from build123d import *

# Parameters (mm, degrees)
F0_W      = 100
F0_H      = 100
F1_DEPTH  = 20
F2_W      = 100
F2_H      = 80
F3_DEPTH  = 20
F4_W      = 30
F4_H      = 80
F5_DEPTH  = 80
F6_R      = 20
F7_R      = 15
F8_DEPTH  = 20
F9_W      = 40
F9_H      = 40
F10_DEPTH = 20
F11_SIZE  = 79.99999


# Not quite as in the source:
# - a fillet or chamfer is up to 0.001 mm smaller than in the source, because OpenCascade refuses the exact size


with BuildPart() as f1:
    # F0 (on Top) → F1 (new body)
    with BuildSketch(Plane.XY):
        with Locations((0.1719114778, -50)):
            Rectangle(F0_W, F0_H)
    extrude(amount=F1_DEPTH)

    # F2 (on Front) → F3 (join)
    with BuildSketch(Plane.XZ):
        with Locations((0.1466497779, 59.8839402659)):
            Rectangle(F2_W, F2_H)
    extrude(amount=F3_DEPTH)

    # F4 (on face) → F5 (join)
    with BuildSketch(Plane.XY.offset(20)):
        with Locations((35.1466497779, -60)):
            Rectangle(F4_W, F4_H)
    extrude(amount=F5_DEPTH)

    # F6
    f6_edges = [f1.edges().sort_by_distance(p)[0] for p in [
        (-49.828089, -100, 10),
    ]]
    fillet(f6_edges, radius=F6_R)

    # F7 (on face) → F8 (cut)
    with BuildSketch(Plane.XY.offset(20)):
        with Locations((-25.480100885, -75)):
            Circle(F7_R)
    extrude(amount=-F8_DEPTH, mode=Mode.SUBTRACT)

    # F9 (on face) → F10 (cut)
    with BuildSketch(Plane.XZ.offset(20)):
        with Locations((-13.2386269793, 61.6098302603)):
            Rectangle(F9_W, F9_H)
    extrude(amount=-F10_DEPTH, mode=Mode.SUBTRACT)

    # F11 (size 80 in the source; OpenCascade refuses exactly that, so slightly less here)
    f11_edges = [f1.edges().sort_by_distance(p)[0] for p in [
        (35.14665, -100, 100),
    ]]
    chamfer(f11_edges, length=F11_SIZE)


solid = f1.part
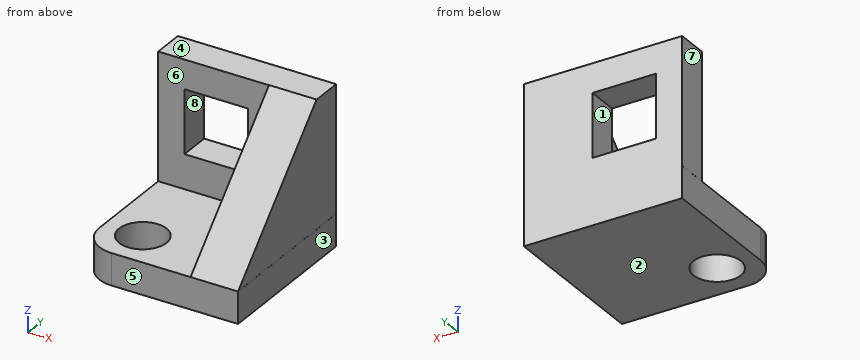
Part model, mm, in its own coordinate system. Face numbers are marked on the shaded views. A direction names the side the tool comes from. Coordinates: 2 decimals unless noted, no trailing zeros. Order: outer loops, then holes, each group sorted by start corner. A loop starts at its lowest first (then second) coordinate and runs counter-clockwise, first axis right, second up.
(1) Pin check, flat tips, straight feed: pin 1 Ø8 at (y, z) = (-87, 19) entering from -X; pin 2 Ø10 at (x, z) = (-36.5, 47) entering from -Y; pin 3 Ø1 at (x, y) = (37, -77) entering from +Z. Stop position of each tip, or through.
Check sheet entries:
pin 1: stops at x = -49.6
pin 2: stops at y = -20
pin 3: stops at z = 43.5
(2) Tool access for the marked faces 4, 5, 6, 7 and 8: list every direction of +Z, -Z, +X, -X, +Y, -Y with a clear straight run to the whole face (end or side of a thin tool).
Check sheet entries:
face 4: +Z, +X, -X, +Y
face 5: +Z, -Z, +X, -X, -Y
face 6: +Z, -X, -Y
face 7: +Z, -Z, -X, +Y, -Y
face 8: +Y, -Y
(3) Slice it at A-A, the plane x = -4.5. Write the cut outline in (y, z), and give its area (3 significant figures).
Check sheet entries:
outline: (-100, 0) - (0, 0) - (0, 41.61) - (-20, 41.61) - (-20, 20) - (-100, 20) - close; (-20, 81.61) - (0, 81.61) - (0, 99.88) - (-20, 99.88) - close
area: 2,800 mm2
(4) Probe L1, parallel to X at y = -25.5, z = 59; L2, parallel to Z at x = -32, y = -8; L3, parallel to Z at x = 15.5, y = -85. List the from-to ranges inside material, lowest first.
Check sheet entries:
L1: x = 20.15 to 50.15
L2: z = 0 to 41.61, 81.61 to 99.88
L3: z = 0 to 20
(5) Slice it at C-C, the plane z = 64.5. Write the cut outline in (x, y).
Check sheet entries:
outline: (-49.85, -20) - (-33.24, -20) - (-33.24, 0) - (-49.85, 0) - close; (6.76, -20) - (20.15, -20) - (20.15, -55.5) - (50.15, -55.5) - (50.15, 0) - (6.76, 0) - close
(6) Slice it at B-B, the plane z = 13.5. Write the cut outline in (x, y), and give its area (3 significant figures).
Check sheet entries:
outline: (-49.83, -80) arc R20 ccw to (-29.83, -100) - (50.17, -100) - (50.17, 0) - (-49.83, 0) - close; hole circle Ø30 at (-25.48, -75)
area: 9,210 mm2
(7) Pull direction Z, two halves, no side cores. Call the marked faces 1, 2 and 3: pulls with the +Z half, pulls with the -Z half, needs draft (parallel to the pull), parting line crosses it, or undercut.
Check sheet entries:
face 1: undercut
face 2: pulls with the -Z half
face 3: needs draft
